For this review, take the finished solid that the model builds, in its own axes (mm). A direction names the side the tool comes from. Round coordinates to 2 decimals unless told otherwise and drop trailing zeros. Write each loop counter-clockwise with the first axis right and the second up, starting at its lowest first coordinate (ties: lowest second). Pieces come first, ordered by that corner, then holes. Notation, with made-up numbers: (-36.5, 50.25) -> (-22.5, 50.25) arc R28 cw to (-22.5, 69.25) -> close; hole circle Ø8 at (40.5, 69.25). An arc over 180 degrees is marked (long way). Write each question's results on one line, items separated by ' | '. Start each with the question number.
Item 1: Clearance check with flat-ended pins moving along their axes: pin 1 (4.5 mm diameter, centred on y = -7, z = 16.2, fed in from -X); pin 2 (2 mm diameter, centred on x = -123.5, z = 42, fed in from +Y). State where each tip first meets the part, or that it passes through.
Item 2: Add section B-B (z = 70). State the section outline as (x, y) points, plus the area to 3 significant figures.
Item 3: Add section C-C (x = -130). State the section outline as (y, z) points.
Item 4: To check wall thickness, follow line 1 along X through (y, z) = (-20.5, 25); line 2 along Y through (x, z) = (-2.2, 31.2); line 3 along Y through (x, z) = (-180, 56). State the ranges of each line that lie inside material, in increasing order.
Item 5: Tool access review of faces 1 (the cylindrical face through (-2.5, -6.9, 63.7)), 2 (the flat face through (-5, -37, 46)), 3 (the cylindrical face through (-307.5, -6.9, 43.7)): name each direction out of +Z, -Z, +X, -X, +Y, -Y from which nothing blocks a thin tool from reaching the whole face with its end or side.
Item 6: Add section A-A (y = -32.5). State the section outline as (x, z) points, plus the area to 3 significant figures.
Item 7: The part is to be moulded in two halves that separate along Z. For faces 4 (the cylindrical face through (-307.715, -77.833, 45.553)), 5 (the cylindrical face through (-2.465, -6.249, 28.815)), 6 (the flat face through (-154.3, -75.4, 92.4)), say which applies: +Z half, -Z half, draft (parallel to the pull), parting line (faces both ways), or undercut.
from build123d import *

# Parameters (mm, degrees)
BASE_FLANGE1_DEPTH = 92.4
SKETCH6_R          = 2.5
CUT_EXTRUDE1_DEPTH = 10
SKETCH7_R          = 2.5
CUT_EXTRUDE2_DEPTH = 10


# Sheet-metal steps are written as plain solids
with BuildPart() as part:
    # Sketch1 → Base-Flange1 (new body)
    with BuildSketch(Plane.XY):
        with BuildLine():
            Line((0, 0), (0, -72.4))
            ThreePointArc((0, -72.4), (-2.225988463, -77.774011537), (-7.6, -80))
            Line((-7.6, -80), (-130, -80))
            Line((-130, -80), (-230, -80))
            Line((-230, -80), (-302.4, -80))
            ThreePointArc((-302.4, -80), (-307.774011537, -77.774011537), (-310, -72.4))
            Line((-310, -72.4), (-310, 0))
            Line((-310, 0), (-305, 0))
            Line((-305, 0), (-305, -72.4))
            ThreePointArc((-305, -72.4), (-304.238477631, -74.238477631), (-302.4, -75))
            Line((-302.4, -75), (-230, -75))
            Line((-230, -75), (-130, -75))
            Line((-130, -75), (-7.6, -75))
            ThreePointArc((-7.6, -75), (-5.761522369, -74.238477631), (-5, -72.4))
            Line((-5, -72.4), (-5, 0))
            Line((-5, 0), (0, 0))
        make_face()
    extrude(amount=BASE_FLANGE1_DEPTH)

    # Sketch6 → Cut-Extrude1 (cut)
    with BuildSketch(Plane(origin=(0, 0, 0), x_dir=(0, 0, -1), z_dir=(1, 0, 0))):
        with Locations((-61.2, -7)):
            Circle(SKETCH6_R)
        with Locations((-31.2, -7)):
            Circle(SKETCH6_R)
    extrude(amount=-CUT_EXTRUDE1_DEPTH, mode=Mode.SUBTRACT)

    # Sketch7 → Cut-Extrude2 (cut)
    with BuildSketch(Plane.ZY.offset(310)):
        with Locations((46.2, -7)):
            Circle(SKETCH7_R)
        with Locations((16.2, -7)):
            Circle(SKETCH7_R)
    extrude(amount=-CUT_EXTRUDE2_DEPTH, mode=Mode.SUBTRACT)


solid = part.part
Responses:
1) pin 1: stops at x = -5 | pin 2: stops at y = -75
2) outline: (-310, -72.4) arc R7.6 ccw to (-302.4, -80) -> (-7.6, -80) arc R7.6 ccw to (0, -72.4) -> (0, 0) -> (-5, 0) -> (-5, -72.4) arc R2.6 cw to (-7.6, -75) -> (-302.4, -75) arc R2.6 cw to (-305, -72.4) -> (-305, 0) -> (-310, 0) -> close | area: 2,280 mm^2
3) outline: (-80, 0) -> (-75, 0) -> (-75, 92.4) -> (-80, 92.4) -> close
4) line 1: x = -310 to -305, -5 to 0 | line 2: y = -77.75 to -9.5, -4.5 to 0 | line 3: y = -80 to -75
5) face 1: +X | face 2: +Z, -Z, +Y | face 3: -X
6) outline: (-310, 0) -> (-305, 0) -> (-305, 92.4) -> (-310, 92.4) -> close; (-5, 0) -> (0, 0) -> (0, 92.4) -> (-5, 92.4) -> close | area: 924 mm^2
7) face 4: draft | face 5: undercut | face 6: +Z half
